Design review of the part built by this model. Coordinates are the model's own, in mm. Face numbers are marked on the shaded views. Give positions to 0.01 mm unless a question says otherwise; leave off trailing zeros. Order: outer loops, then holes, each group sorted by start corner. A loop starts at its lowest first (then second) coordinate and runs counter-clockwise, first axis right, second up. Notation, with made-up numbers: (-27.75, 46) - (-23.75, 46) arc R14 ccw to (-23.75, 53) - close; hole circle Ø8 at (29, 16.25). An arc over 180 degrees is marked (long way). Write each question's results on one line, items separated by ' | '. Start each with the question number.
```python
from build123d import *

# Parameters (mm, degrees)
ESBO_O1_R                = 3
ESBO_O1_W                = 2
ESBO_O1_H                = 16
RESSALTO_EXTRUS_O1_DEPTH = 2


with BuildPart() as part:
    # Esboço1 → Ressalto-extrusão1 (new body)
    with BuildSketch(Plane.XY):
        with BuildLine():
            Line((-21.07, 11), (0, 9))
            ThreePointArc((0, 9), (8.911247748, 1.260818614), (2.496770452, -8.646741427))
            add(Edge.make_bspline(
                [(-65.07, -13), (-43.239788601, -19.093527225), (-19.750123263, -17.642441034), (2.496770452, -8.646741427)],
                knots=[0, 0, 0, 0, 0.972962774, 0.972962774, 0.972962774, 0.972962774], degree=3))
            Line((-65.07, -13), (-87.07, -13))
            Line((-87.07, -13), (-87.07, 13))
            Line((-87.07, 13), (-72.07, 13))
            Line((-72.07, 13), (-52.07, 11))
            Line((-52.07, 11), (-44.07, 11))
            Line((-44.07, 11), (-44.07, -7.5))
            Line((-44.07, -7.5), (-21.07, -7.5))
            Line((-21.07, -7.5), (-21.07, 11))
        make_face()
        Circle(ESBO_O1_R, mode=Mode.SUBTRACT)
        with BuildLine():
            Line((-52.07, 2.107200462), (-52.07, -3.107200462))
            ThreePointArc((-52.07, -3.107200462), (-52.32404099, -3.773192321), (-52.957090312, -4.100805717))
            Line((-52.957090312, -4.100805717), (-72.957090312, -6.37353299))
            ThreePointArc((-72.957090312, -6.37353299), (-73.735991859, -6.125886745), (-74.07, -5.379927735))
            Line((-74.07, -5.379927735), (-74.07, 4.379927735))
            ThreePointArc((-74.07, 4.379927735), (-73.735991859, 5.125886745), (-72.957090312, 5.37353299))
            Line((-72.957090312, 5.37353299), (-52.957090312, 3.100805717))
            ThreePointArc((-52.957090312, 3.100805717), (-52.32404099, 2.773192321), (-52.07, 2.107200462))
        make_face(mode=Mode.SUBTRACT)
        with Locations((-83.07, 0)):
            Rectangle(ESBO_O1_W, ESBO_O1_H, mode=Mode.SUBTRACT)
    extrude(amount=RESSALTO_EXTRUS_O1_DEPTH)


solid = part.part
```
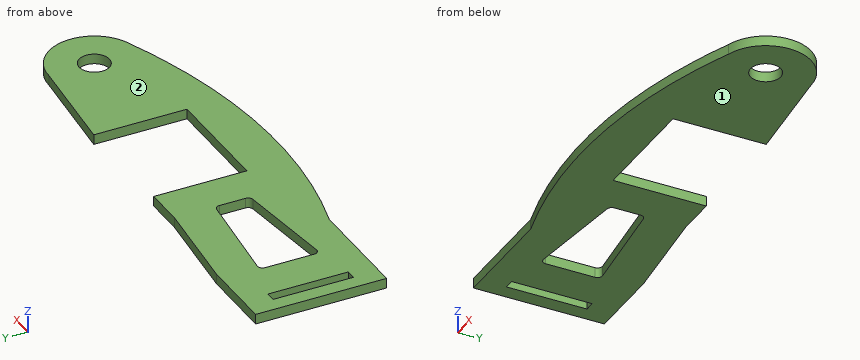
Q1. For line 1 (X direction, y = 1.25, z = 1.05); line 2 (X direction, y = 6.5, z = 0.15); line 3 (X direction, y = 1.5, z = 0.1), list the stretches that pass through material, from the lowest coordinate up. Write a range as [from, to].
Q2. Draft analysis for pull direction Z (two halves, no side actions). For the marked faces 1 and 2, state which applies: pulls with the +Z half, pulls with the -Z half, needs draft (parallel to the pull), parting line crosses it, or undercut.
Q3. Add section B-B (z = 0.95). Give the number of separate pieces and of enclosed holes in the cut face, plus the area to 3 significant figures.
Q4. Add section A-A (y = 0). Give the boundary of the cut face in (x, z).
Q5. Insertion check: pin 1 Ø6 at (x, y) = (-51, -5) entering from -Z; pin 2 Ø0.6 at (y, z) = (2, 1.5) entering from +X; pin 3 Ø1 at (x, z) = (-41.5, 0.5) entering from -Y; pin 4 Ø1 at (x, z) = (-83.5, 1) entering from -Y. Each pin has a flat end and moves straight along its axis. Give the tip position at first contact, or say it passes through.
Verdict:
1) line 1: x = [-87.07, -84.07], [-82.07, -74.07], [-52.07, -44.07], [-21.07, -2.73], [2.73, 8.91] | line 2: x = [-87.07, -84.07], [-82.07, -44.07], [-21.07, 6.22] | line 3: x = [-87.07, -84.07], [-82.07, -74.07], [-52.07, -44.07], [-21.07, -2.6], [2.6, 8.87]
2) face 1: pulls with the -Z half | face 2: pulls with the +Z half
3) separate pieces: 1 | enclosed holes: 3 | area: 1,670 mm2
4) outline: (-87.07, 0) - (-84.07, 0) - (-84.07, 2) - (-87.07, 2) - close; (-82.07, 0) - (-74.07, 0) - (-74.07, 2) - (-82.07, 2) - close; (-52.07, 0) - (-44.07, 0) - (-44.07, 2) - (-52.07, 2) - close; (-21.07, 0) - (-3, 0) - (-3, 2) - (-21.07, 2) - close; (3, 0) - (9, 0) - (9, 2) - (3, 2) - close
5) pin 1: stops at z = 0 | pin 2: stops at x = 8.84 | pin 3: stops at y = -16.65 | pin 4: stops at y = -13
